from build123d import *

# Parameters (mm, degrees)
F0_W     = 40.0103181601
F0_H     = 24.0946123376
F1_DEPTH = 7.62


with BuildPart() as f1:
    # F0 (on Top) → F1 (new body)
    with BuildSketch(Plane.XY):
        with Locations((-0.1676287502, 3.8467827253)):
            Rectangle(F0_W, F0_H)
        with BuildLine():
            Line((-11.7563733071, 0.7942912366), (-10.7646722607, 6.4043121633))
            Line((-10.7646722607, 6.4043121633), (-11.5619816778, 6.5273256163))
            Line((-11.5619816778, 6.5273256163), (-11.5133837704, 6.7794272605))
            Line((-11.5133837704, 6.7794272605), (-6.7401580604, 6.7794272605))
            Line((-6.7401580604, 6.7794272605), (-7.0104839199, 5.2561866028))
            Line((-7.0104839199, 5.2561866028), (-7.3233329483, 5.2561866028))
            Line((-7.3233329483, 5.2561866028), (-7.2944779408, 6.2858547642))
            add(Edge.make_bspline(
                [(-7.2944779408, 6.2858547642), (-7.8123493908, 6.3511582022), (-8.8177185985, 6.3511582022)],
                knots=[0, 0, 0, 1, 1, 1], degree=2))
            Line((-8.8177185985, 6.3511582022), (-9.8580175522, 6.3511582022))
            Line((-9.8580175522, 6.3511582022), (-10.2984360873, 3.8650715056))
            Line((-10.2984360873, 3.8650715056), (-8.5808038003, 3.8650715056))
            Line((-8.5808038003, 3.8650715056), (-8.2968097794, 4.6244138076))
            Line((-8.2968097794, 4.6244138076), (-7.9930728586, 4.6244138076))
            Line((-7.9930728586, 4.6244138076), (-8.3393329483, 2.6683480378))
            Line((-8.3393329483, 2.6683480378), (-8.6430698691, 2.6683480378))
            Line((-8.6430698691, 2.6683480378), (-8.6521819767, 3.4383211319))
            Line((-8.6521819767, 3.4383211319), (-10.3698142637, 3.4383211319))
            Line((-10.3698142637, 3.4383211319), (-10.8299756987, 0.8413704593))
            Line((-10.8299756987, 0.8413704593), (-9.5770609005, 0.8413704593))
            add(Edge.make_bspline(
                [(-9.5770609005, 0.8413704593), (-8.3621132174, 0.8413704593), (-7.9596617973, 0.9173046895)],
                knots=[0, 0, 0, 1, 1, 1], degree=2))
            Line((-7.9596617973, 0.9173046895), (-7.4797574625, 2.0942852575))
            Line((-7.4797574625, 2.0942852575), (-7.1669084341, 2.0942852575))
            Line((-7.1669084341, 2.0942852575), (-7.5556916927, 0.4146200856))
            Line((-7.5556916927, 0.4146200856), (-12.6341730081, 0.4146200856))
            Line((-12.6341730081, 0.4146200856), (-12.5870937854, 0.6667217299))
            Line((-12.5870937854, 0.6667217299), (-11.7563733071, 0.7942912366))
        make_face(mode=Mode.SUBTRACT)
        with BuildLine():
            add(Edge.make_bspline(
                [(-1.5644809304, 0.8102374249), (-2.3830519319, 0.3189429556), (-3.437019047, 0.3189429556)],
                knots=[0, 0, 0, 1, 1, 1], degree=2))
            add(Edge.make_bspline(
                [(-3.437019047, 0.3189429556), (-4.2009174027, 0.3189429556), (-4.8106692712, 0.639385407)],
                knots=[0, 0, 0, 1, 1, 1], degree=2))
            add(Edge.make_bspline(
                [(-4.8106692712, 0.639385407), (-5.4204211396, 0.9598278584), (-5.7575691217, 1.5437620886)],
                knots=[0, 0, 0, 1, 1, 1], degree=2))
            add(Edge.make_bspline(
                [(-5.7575691217, 1.5437620886), (-6.0947171038, 2.1276963188), (-6.0947171038, 2.8536275595)],
                knots=[0, 0, 0, 1, 1, 1], degree=2))
            add(Edge.make_bspline(
                [(-6.0947171038, 2.8536275595), (-6.0947171038, 3.9971970662), (-5.6201281651, 4.9251133592)],
                knots=[0, 0, 0, 1, 1, 1], degree=2))
            add(Edge.make_bspline(
                [(-5.6201281651, 4.9251133592), (-5.1455392263, 5.8530296521), (-4.3246901979, 6.3519175445)],
                knots=[0, 0, 0, 1, 1, 1], degree=2))
            add(Edge.make_bspline(
                [(-4.3246901979, 6.3519175445), (-3.5038411695, 6.8508054369), (-2.4498740544, 6.8508054369)],
                knots=[0, 0, 0, 1, 1, 1], degree=2))
            add(Edge.make_bspline(
                [(-2.4498740544, 6.8508054369), (-1.6859756987, 6.8508054369), (-1.0762238302, 6.5303629855)],
                knots=[0, 0, 0, 1, 1, 1], degree=2))
            add(Edge.make_bspline(
                [(-1.0762238302, 6.5303629855), (-0.4664719618, 6.209920534), (-0.1293239797, 5.6282643308)],
                knots=[0, 0, 0, 1, 1, 1], degree=2))
            add(Edge.make_bspline(
                [(-0.1293239797, 5.6282643308), (0.2078240024, 5.0466081275), (0.2078240024, 4.316120833)],
                knots=[0, 0, 0, 1, 1, 1], degree=2))
            add(Edge.make_bspline(
                [(0.2078240024, 4.316120833), (0.2078240024, 3.1907755415), (-0.2690429633, 2.2461537179)],
                knots=[0, 0, 0, 1, 1, 1], degree=2))
            add(Edge.make_bspline(
                [(-0.2690429633, 2.2461537179), (-0.7459099289, 1.3015318943), (-1.5644809304, 0.8102374249)],
                knots=[0, 0, 0, 1, 1, 1], degree=2))
        make_face(mode=Mode.SUBTRACT)
        Polygon((2.8655220592, 0.4146200856), (0.3308374553, 0.4146200856), (0.3688045704, 0.6667217299), (1.2040811025, 0.7942912366), (2.1866700412, 6.4043121633), (1.3984727318, 6.5273256163), (1.4364398469, 6.7794272605), (3.9863112968, 6.7794272605), (3.9483441817, 6.5273256163), (3.0978808036, 6.4043121633), (2.6620183222, 3.9030386207), (5.6568643611, 3.9030386207), (6.0927268424, 6.4043121633), (5.304529533, 6.5273256163), (5.3424966481, 6.7794272605), (7.8908494134, 6.7794272605), (7.8528822983, 6.5273256163), (7.0084936586, 6.4043121633), (6.0259047199, 0.7942912366), (6.8141020293, 0.6667217299), (6.7715788604, 0.4146200856), (4.2277821488, 0.4146200856), (4.2657492639, 0.6667217299), (5.1101379037, 0.7942912366), (5.5809301309, 3.476288247), (2.586084092, 3.476288247), (2.1152918648, 0.7942912366), (2.9034891743, 0.6667217299), align=None, mode=Mode.SUBTRACT)
        with BuildLine():
            Line((7.5688882774, 0.7608801753), (7.8164338678, 2.1747755415))
            Line((7.8164338678, 2.1747755415), (8.1247268424, 2.1747755415))
            Line((8.1247268424, 2.1747755415), (8.1292828962, 1.2696395176))
            add(Edge.make_bspline(
                [(8.1292828962, 1.2696395176), (8.2857074104, 1.0312060348), (8.6631005345, 0.8679474399)],
                knots=[0, 0, 0, 1, 1, 1], degree=2))
            add(Edge.make_bspline(
                [(8.6631005345, 0.8679474399), (9.0404936586, 0.704688845), (9.4626879784, 0.704688845)],
                knots=[0, 0, 0, 1, 1, 1], degree=2))
            add(Edge.make_bspline(
                [(9.4626879784, 0.704688845), (10.2402544956, 0.704688845), (10.6609301309, 1.0722105191)],
                knots=[0, 0, 0, 1, 1, 1], degree=2))
            add(Edge.make_bspline(
                [(10.6609301309, 1.0722105191), (11.0816057662, 1.4397321932), (11.0816057662, 2.0988413113)],
                knots=[0, 0, 0, 1, 1, 1], degree=2))
            add(Edge.make_bspline(
                [(11.0816057662, 2.0988413113), (11.0816057662, 2.3554990094), (10.9677044209, 2.5453345849)],
                knots=[0, 0, 0, 1, 1, 1], degree=2))
            add(Edge.make_bspline(
                [(10.9677044209, 2.5453345849), (10.8538030756, 2.7351701603), (10.6639675001, 2.8870386207)],
                knots=[0, 0, 0, 1, 1, 1], degree=2))
            add(Edge.make_bspline(
                [(10.6639675001, 2.8870386207), (10.4741319246, 3.0389070811), (10.2341797572, 3.1672359302)],
                knots=[0, 0, 0, 1, 1, 1], degree=2))
            add(Edge.make_bspline(
                [(10.2341797572, 3.1672359302), (9.9942275898, 3.2955647792), (9.7428852879, 3.4261716551)],
                knots=[0, 0, 0, 1, 1, 1], degree=2))
            add(Edge.make_bspline(
                [(9.7428852879, 3.4261716551), (9.4915429859, 3.5567785311), (9.2515908185, 3.7063689645)],
                knots=[0, 0, 0, 1, 1, 1], degree=2))
            add(Edge.make_bspline(
                [(9.2515908185, 3.7063689645), (9.0116386511, 3.855959398), (8.8218030756, 4.0526290542)],
                knots=[0, 0, 0, 1, 1, 1], degree=2))
            add(Edge.make_bspline(
                [(8.8218030756, 4.0526290542), (8.6319675001, 4.2492987104), (8.5180661548, 4.5059564085)],
                knots=[0, 0, 0, 1, 1, 1], degree=2))
            add(Edge.make_bspline(
                [(8.5180661548, 4.5059564085), (8.4041648095, 4.7626141065), (8.4041648095, 5.1088741962)],
                knots=[0, 0, 0, 1, 1, 1], degree=2))
            add(Edge.make_bspline(
                [(8.4041648095, 5.1088741962), (8.4041648095, 5.953262836), (8.9782275898, 6.4020341364)],
                knots=[0, 0, 0, 1, 1, 1], degree=2))
            add(Edge.make_bspline(
                [(8.9782275898, 6.4020341364), (9.5522903701, 6.8508054369), (10.6199256466, 6.8508054369)],
                knots=[0, 0, 0, 1, 1, 1], degree=2))
            add(Edge.make_bspline(
                [(10.6199256466, 6.8508054369), (11.4369779635, 6.8508054369), (12.1583531503, 6.670081969)],
                knots=[0, 0, 0, 1, 1, 1], degree=2))
            Line((12.1583531503, 6.670081969), (11.9259944059, 5.3457889944))
            Line((11.9259944059, 5.3457889944), (11.6177014314, 5.3457889944))
            Line((11.6177014314, 5.3457889944), (11.5934024777, 6.1567665729))
            add(Edge.make_bspline(
                [(11.5934024777, 6.1567665729), (11.4415340173, 6.2812987104), (11.1712081578, 6.3663450482)],
                knots=[0, 0, 0, 1, 1, 1], degree=2))
            add(Edge.make_bspline(
                [(11.1712081578, 6.3663450482), (10.9008822983, 6.4513913861), (10.5500661548, 6.4513913861)],
                knots=[0, 0, 0, 1, 1, 1], degree=2))
            add(Edge.make_bspline(
                [(10.5500661548, 6.4513913861), (9.9182933596, 6.4513913861), (9.5765893237, 6.1430984115)],
                knots=[0, 0, 0, 1, 1, 1], degree=2))
            add(Edge.make_bspline(
                [(9.5765893237, 6.1430984115), (9.2348852879, 5.8348054369), (9.2348852879, 5.2789668719)],
                knots=[0, 0, 0, 1, 1, 1], degree=2))
            add(Edge.make_bspline(
                [(9.2348852879, 5.2789668719), (9.2348852879, 4.9797860049), (9.4482604747, 4.7329997568)],
                knots=[0, 0, 0, 1, 1, 1], degree=2))
            add(Edge.make_bspline(
                [(9.4482604747, 4.7329997568), (9.6616356616, 4.4862135086), (10.0838299814, 4.2735976641)],
                knots=[0, 0, 0, 1, 1, 1], degree=2))
            add(Edge.make_bspline(
                [(10.0838299814, 4.2735976641), (10.7292709381, 3.936449682), (11.0140243013, 3.7610416103)],
                knots=[0, 0, 0, 1, 1, 1], degree=2))
            add(Edge.make_bspline(
                [(11.0140243013, 3.7610416103), (11.2987776645, 3.5856335385), (11.4908912669, 3.3859265131)],
                knots=[0, 0, 0, 1, 1, 1], degree=2))
            add(Edge.make_bspline(
                [(11.4908912669, 3.3859265131), (11.6830048693, 3.1862194877), (11.7999435838, 2.9303211319)],
                knots=[0, 0, 0, 1, 1, 1], degree=2))
            add(Edge.make_bspline(
                [(11.7999435838, 2.9303211319), (11.9168822983, 2.6744227762), (11.9168822983, 2.3418308479)],
                knots=[0, 0, 0, 1, 1, 1], degree=2))
            add(Edge.make_bspline(
                [(11.9168822983, 2.3418308479), (11.9168822983, 1.363797963), (11.2782754224, 0.8413704593)],
                knots=[0, 0, 0, 1, 1, 1], degree=2))
            add(Edge.make_bspline(
                [(11.2782754224, 0.8413704593), (10.6396685465, 0.3189429556), (9.433832971, 0.3189429556)],
                knots=[0, 0, 0, 1, 1, 1], degree=2))
            add(Edge.make_bspline(
                [(9.433832971, 0.3189429556), (8.835471237, 0.3189429556), (8.3586042714, 0.4404377239)],
                knots=[0, 0, 0, 1, 1, 1], degree=2))
            add(Edge.make_bspline(
                [(8.3586042714, 0.4404377239), (7.8817373058, 0.5619324922), (7.5688882774, 0.7608801753)],
                knots=[0, 0, 0, 1, 1, 1], degree=2))
        make_face(mode=Mode.SUBTRACT)
    extrude(amount=F1_DEPTH)


solid = f1.part
Read the model definition and answer for the solid it produces. Units are mm, in the model's axes. A direction names the side the tool comes from. Round coordinates to 2 decimals unless told otherwise and drop trailing zeros. One line per question, with ' | ' between items. Start each with the question number.
1. Section A-A (z = 5.25) is taken. Give the number of separate pieces and of enclosed holes in the cut face, and give its area (3 significant figures).
2. Find the intervals of material crossed by probe 1 along Y at (x, z) = (-9.5, 2.5); probe 2 along Y at (x, z) = (-12, 2.75); probe 3 along Y at (x, z) = (5, 0.5), in increasing order. Write a range as [from, to].
3. For faces 1 (the face through (-7.359, 1.266, 3.757)), 2 (the face through (-20.173, 4, 4)), determine the directions among +Z, -Z, +X, -X, +Y, -Y from which every point of the face is accessible in a straight line to the end or side of a thin tool.
4. For a pull along X with two mould halves and no side action, classify faces 3 (the face through (-10.075, 5.126, 3.757)), 4 (the face through (0, -8.201, 4)), 5 (the face through (19.838, 4, 4)) as +X half, -X half, draft (parallel to the pull), parting line (faces both ways), or undercut.
Filled in:
1) separate pieces: 1 | enclosed holes: 4 | area: 895 mm²
2) probe 1: [-8.2, 0.41], [0.84, 3.44], [3.87, 6.35], [6.78, 15.89] | probe 2: [-8.2, 0.41], [0.76, 15.89] | probe 3: [-8.2, 0.41], [0.78, 3.48], [3.9, 15.89]
3) face 1: +Z, -Z | face 2: +Z, -Z, -X, +Y, -Y
4) face 3: undercut | face 4: draft | face 5: +X half
